Autodesk Inventor part; units mm, degrees
ref_plane "YZ Plane" through (0, 0, 0) normal (1, 0, 0) x (0, 1, 0)
ref_plane "XZ Plane" through (0, 0, 0) normal (0, 1, 0) x (-1, 0, 0)
ref_plane "XY Plane" through (0, 0, 0) normal (0, 0, 1) x (1, 0, 0)
sketch "Sketch1" plane through (0, 0, 0) normal (0, 1, 0) x (-1, 0, 0)
  line L0 (0, 0) -> (-20, 0)
  line L1 (-20, 0) -> (-20, -20)
  line L2 (-20, -20) -> (0, -20)
  line L3 (0, -20) -> (0, 0)
  dimension "d0" = 20
  dimension "d1" = 20
extrude "Extrusion1" add sketch "Sketch1" along normal blind 4
sketch "Sketch2" plane through (0, 4, 0) normal (0, 1, 0) x (1, 0, 0)
  line L0 (0, 0) -> (20, 0)
  line L1 (20, 0) -> (20, 4)
  line L2 (20, 4) -> (4, 4)
  line L3 (0, 4) -> (0, 0)
  line L4 (0, 0) -> (4, 0)
  line L5 (4, 20) -> (0, 20)
  line L6 (0, 20) -> (0, 0)
  line L7 (4, 4) -> (4, 20)
  line L8 (0, 0) -> (20, 0)
  line L9 (0, 0) -> (20, 0)
  line L10 (0, 20) -> (0, 0)
  line L11 (0, 0) -> (0, 20)
extrude "Extrusion2" add sketch "Sketch2" along normal blind 16
hole "Hole2" at (12, 12, -4) direction (0, 0, 1) diameter 4 end through all
hole "Hole3" at (4, 12, -12) direction (-1, 0, 0) diameter 4 end through all
chamfer "Chamfer1" distance 12 angle 45 1 edges at (20, 2, -20)
chamfer "Chamfer2" distance 4 angle 45 1 edges at (20, 20, -2)
chamfer "Chamfer3" distance 4 angle 45 1 edges at (2, 20, -20)
sketch "Sketch3" plane through (20, 4, -4) normal (0, 0, -1) x (-1, 0, 0)
  line L0 (8, 12.0415) -> (11.5, 10.0207)
  line L1 (11.5, 10.0207) -> (11.5, 5.9793)
  line L2 (11.5, 5.9793) -> (8, 3.9585)
  line L3 (8, 3.9585) -> (4.5, 5.9793)
  line L4 (4.5, 5.9793) -> (4.5, 10.0207)
  line L5 (4.5, 10.0207) -> (8, 12.0415)
  point P0 (20, -4)
  point P1 (8, 8)
  dimension "d51" = 7
sketch "Sketch4" plane through (4, 4, -4) normal (1, 0, 0) x (0, 0, -1)
  line L0 (3.9585, 8) -> (5.9793, 11.5)
  line L1 (5.9793, 11.5) -> (10.0207, 11.5)
  line L2 (10.0207, 11.5) -> (12.0415, 8)
  line L3 (12.0415, 8) -> (10.0207, 4.5)
  line L4 (10.0207, 4.5) -> (5.9793, 4.5)
  line L5 (5.9793, 4.5) -> (3.9585, 8)
  point P0 (-4, -4)
  point P1 (8, 8)
  dimension "d52" = 7
extrude "Extrusion3" cut sketch "Sketch3" against normal blind 2
extrude "Extrusion4" cut sketch "Sketch4" against normal blind 2
properties part number "Frame2WayBlock" material "PLA Orange"
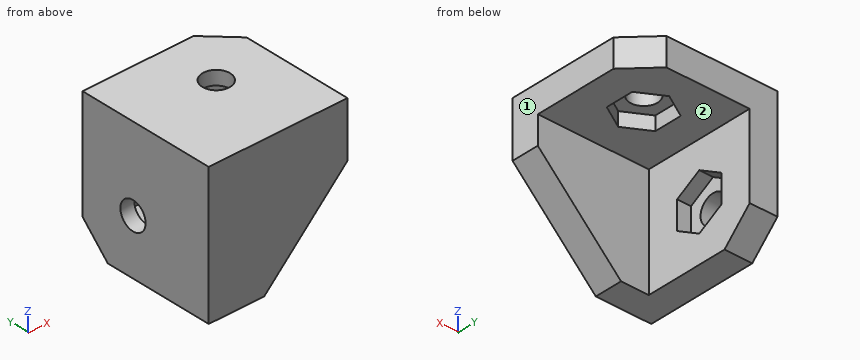
Verification items for the finished model (mm, model axes). Face numbers are marked on the shaded views. A direction names the side the tool comes from. Round coordinates to 2 decimals unless told otherwise and drop trailing zeros. Order: outer loops, then holes, each group sorted by start corner. A loop starts at its lowest first (then second) coordinate and runs counter-clockwise, first axis right, second up. Notation, with made-up numbers: (-28, -35) - (25, -35) arc R8 cw to (25, -28) - close; hole circle Ø11 at (-23, -18). An arc over 180 degrees is marked (long way). Use CSV: the item, a comma, the result in double quotes. Start each with the question number.
1) Section check D-D, the plane x = 11. Record the cut outline in (y, z), plus the area to 3 significant figures.
2) Go/stop test with flat-tipped pins: P1, Ø6, axis at y = 13.5, z = -13, coming from the -X side; P2, Ø7.5, axis at y = 11, z = -13, coming from the +X side; P3, Ø8, axis at x = 15.5, y = 9.5, coming from the -Z side. Record where each tip stops, or that it passes through.
3) Section check A-A, the plane z = -2.5. Record the cut outline in (x, y).
4) Section check C-C, the plane y = 12.5. Record the cut outline in (x, z), plus the area to 3 significant figures.
5) Section check B-B, the plane z = -12. Record the cut outline in (x, y), plus the area to 3 significant figures.
6) Access from +Z, -Z, +X, -X, +Y, -Y to the whole of each face (thin tool, end or side, straight path). Record for the marked faces 1 and 2.
7) Thickness scan on L1, parallel to X at y = 12, z = -0.75; L2, parallel to X at y = 17.75, z = -7.25. Record the ranges inside material, lowest first.
Answers:
1,outline,"(0, -17) - (4, -17) - (4, -4) - (8.54, -4) - (8.54, -2) - (10.27, -2) - (10.27, 0) - (0, 0) - close; (13.73, -2) - (15.46, -2) - (15.46, -4) - (20, -4) - (20, 0) - (13.73, 0) - close"
1,area,"111 mm²"
2,P1,"stops at x = 0"
2,P2,"stops at x = 4"
2,P3,"stops at z = -4"
3,outline,"(0, 0) - (20, 0) - (20, 16) - (16, 20) - (0, 20) - close; hole (8.5, 9.98) - (12, 7.96) - (15.5, 9.98) - (15.5, 14.02) - (12, 16.04) - (8.5, 14.02) - close"
4,outline,"(0, -20) - (4, -20) - (4, -15.75) - (2, -15.75) - (2, -13.94) - (0, -13.94) - close; (0, -10.06) - (2, -10.06) - (2, -8.25) - (4, -8.25) - (4, -4) - (8.5, -4) - (8.5, -2) - (10.06, -2) - (10.06, 0) - (0, 0) - close; (13.94, -2) - (15.5, -2) - (15.5, -4) - (20, -4) - (20, 0) - (13.94, 0) - close"
4,area,"99.5 mm²"
5,outline,"(0, 0) - (16, 0) - (16, 4) - (4, 4) - (4, 8.5) - (2, 8.5) - (2, 10) - (0, 10) - close; (0, 14) - (2, 14) - (2, 15.5) - (4, 15.5) - (4, 20) - (0, 20) - close"
5,area,"106 mm²"
6,face 1,"+Z, -Z, +X, +Y, -Y"
6,face 2,"-Z, +X, +Y"
7,L1,"x = 0 to 10, 14 to 20"
7,L2,"x = 0 to 4"
